Work out the finished part from the listing and answer in its coordinate system (mm). A direction names the side the tool comes from. Coordinates: 2 decimals unless noted, no trailing zeros. Loops run counter-clockwise (first coordinate to the right, second up) from the corner with the lowest first, then second, coordinate; pieces in that order, holes last. Notation, with made-up numbers: (-30, -21.5) - (-12, -21.5) arc R34 ccw to (-12, 15.5) - close; hole circle Ø7 at (-4.75, 82.5). An arc over 180 degrees is marked (long way). Write each question's results on one line, items separated by ' | '. Start each with the question number.
Item 1: Consider probe 1 along X at (y, z) = (-5, 4.75); probe 2 along X at (y, z) = (3, 8); probe 3 along X at (y, z) = (-5, 16.25). Determine where each line is inside the solid, lowest interval first. Write a range as [from, to].
Item 2: Each of these flat-tipped pins is pushed along its axis until it touches: pin 1 Ø4 at (y, z) = (-3.5, 18.5) entering from -X; pin 2 Ø2 at (x, y) = (10, -5) entering from -Z; pin 3 Ø6 at (x, y) = (1, 4.5) entering from -Z. Where does it stop, or does it pass through?
Item 3: Section B-B, the plane y = 3.75 is taken. Write down the section's boundary in (x, z), plus the area to 3 significant figures.
Item 4: Section D-D, the plane x = 12 is taken. Write down the section's boundary in (y, z), plus the area to 3 significant figures.
Item 5: Section C-C, the plane z = 9.25 is taken. Count the separate pieces of the cut face and the enclosed holes in it, plus the area to 3 significant figures.
Item 6: For a pull along Z with two mould halves and no side action, classify faces 3 (the face through (17.71, -3, 11)), 4 (the face through (-6.45, -2.72, 14.02)), 5 (the face through (-7.137, -2.632, 17.774)), 6 (the face through (10.54, -2.93, 7.17)) as +Z half, -Z half, draft (parallel to the pull), parting line (faces both ways), or undercut.
Item 7: Section A-A, the plane y = -2.25 is taken. Write down the section's boundary in (x, z).
Item 8: A tool of negligible diameter and unlimited length cuts with its end or side. For faces 1 (the face through (-5.17, -0.7, 5.4)), 2 (the face through (-10.57, -3, 8)), from which of +Z, -Z, +X, -X, +Y, -Y can it reach the whole face along a straight path? Write none if from no direction.
from build123d import *

# Parameters (mm, degrees)
SKETCH1_W           = 28.28
SKETCH1_H           = 20
BOSS_EXTRUDE1_DEPTH = 40
SKETCH2_W           = 28.28
SKETCH2_H           = 17.86
CUT_EXTRUDE1_DEPTH  = 29
SKETCH3_R           = 2.675
CUT_EXTRUDE2_DEPTH  = 19
CUT_EXTRUDE3_START  = -7
SKETCH4_R           = 5
CUT_EXTRUDE3_DEPTH  = 19


with BuildPart() as part:
    # Sketch1 → Boss-Extrude1 (new body)
    with BuildSketch(Plane.XY):
        with Locations((3.569509613, -2.786541121)):
            Rectangle(SKETCH1_W, SKETCH1_H)
    extrude(amount=BOSS_EXTRUDE1_DEPTH)

    # Sketch2 → Cut-Extrude1 (cut)
    with BuildSketch(Plane.XZ.offset(12.786541121)):
        Polygon((-10.570490387, 0), (3.569509613, 14.14), (17.709509613, 0), align=None)
        with Locations((3.569509613, 31.07)):
            Rectangle(SKETCH2_W, SKETCH2_H)
    extrude(amount=-CUT_EXTRUDE1_DEPTH, mode=Mode.SUBTRACT)

    # Sketch3 → Cut-Extrude2 (cut)
    with BuildSketch(Plane(origin=(-5.285245194, 0, 5.285245194), x_dir=(-0.707106781186544, 0, -0.7071067811865511), z_dir=(0.7071067811865511, 0, -0.707106781186544))):
        with Locations((-2.524024453, -2.786541121)):
            Circle(SKETCH3_R)
    extrude(amount=-CUT_EXTRUDE2_DEPTH, mode=Mode.SUBTRACT)

    # Sketch4 → Cut-Extrude3 (cut)
    with BuildSketch(Plane(origin=(-5.285245194, 0, 5.285245194), x_dir=(-0.707106781186544, 0, -0.7071067811865511), z_dir=(0.7071067811865511, 0, -0.707106781186544)).offset(CUT_EXTRUDE3_START)):
        with Locations((-2.524024453, -2.786541121)):
            Circle(SKETCH4_R)
    extrude(amount=-CUT_EXTRUDE3_DEPTH, mode=Mode.SUBTRACT)


solid = part.part
Answer key:
1) probe 1: x = [-10.57, -5.82], [12.96, 17.71] | probe 2: x = [-10.57, -2.57], [9.71, 17.71] | probe 3: x = [-6.34, 17.71]
2) pin 1: stops at x = -10.02 | pin 2: stops at z = 6.71 | pin 3: stops at z = 8.57
3) outline: (-10.57, 0) - (3.57, 14.14) - (17.71, 0) - (17.71, 22.14) - (-10.57, 22.14) - close | area: 426 mm^2
4) outline: (-12.79, 5.71) - (7.21, 5.71) - (7.21, 22.14) - (-12.79, 22.14) - close | area: 329 mm^2
5) separate pieces: 2 | enclosed holes: 1 | area: 338 mm^2
6) face 3: draft | face 4: undercut | face 5: undercut | face 6: -Z half
7) outline: (-10.57, 0) - (-5.35, 5.22) - (-10.3, 10.17) - (-10.57, 9.9) - close; (-10.57, 21.17) - (-4.94, 15.53) - (-6.6, 13.87) - (-1.65, 8.92) - (3.57, 14.14) - (17.71, 0) - (17.71, 22.14) - (-10.57, 22.14) - close
8) face 1: -Z, +Y, -Y | face 2: +Z, -Z, -X, +Y, -Y
